Can you work these out from the model? Positions are in its coordinate system, mm. Face numbers are marked on the shaded views. A direction names the side the tool comes from. Give positions to 0.01 mm unless a question says otherwise; leave off trailing zeros. Loops run counter-clockwise (first coordinate to the right, second up) from the corner with the lowest first, then second, coordinate; pieces in that order, holes last. Notation, with made-up numbers: (8.5, 19.5) - (56.5, 19.5) arc R22 ccw to (56.5, 28.5) - close; hole circle Ø7 at (-12, 59.5). An arc over 180 degrees is marked (long way). Answer as a JSON object with one key per item and string values.
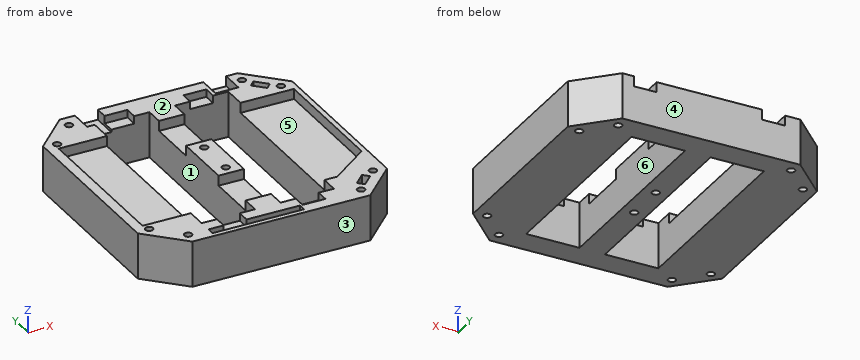
```python
from build123d import *

# Parameters (mm, degrees)
PAD_DEPTH       = 18
SKETCH001_R     = 1.5
POCKET_DEPTH    = 18.001
SKETCH002_W     = 21
SKETCH002_H     = 78
POCKET001_DEPTH = 18.001
SKETCH003_W     = 9
SKETCH003_H     = 88
POCKET002_DEPTH = 3
SKETCH004_W     = 12
SKETCH004_H     = 20
SKETCH004_W_2   = 19
SKETCH004_H_2   = 62
SKETCH004_W_3   = 9
SKETCH004_H_3   = 9
SKETCH004_W_4   = 36
SKETCH004_H_4   = 3
POCKET003_DEPTH = 4
SKETCH005_W     = 6
SKETCH005_H     = 1
POCKET004_DEPTH = 4


with BuildPart() as part:
    # Sketch → Pad (new body)
    with BuildSketch(Plane.XY):
        Polygon((-49, 35), (-35, 49), (35, 49), (49, 35), (49, -35), (35, -49), (-35, -49), (-49, -35), align=None)
    extrude(amount=PAD_DEPTH)

    # Sketch001 (on DatumPlane) → Pocket (cut, through all)
    with BuildSketch(Plane.XY.offset(18)):
        with Locations((-34, 44)):
            Circle(SKETCH001_R)
        with Locations((34, 44)):
            Circle(SKETCH001_R)
        with Locations((44, 34)):
            Circle(SKETCH001_R)
        with Locations((-44, 34)):
            Circle(SKETCH001_R)
        with Locations((-44, -34)):
            Circle(SKETCH001_R)
        with Locations((-34, -44)):
            Circle(SKETCH001_R)
        with Locations((34, -44)):
            Circle(SKETCH001_R)
        with Locations((44, -34)):
            Circle(SKETCH001_R)
        with Locations((0, 8)):
            Circle(SKETCH001_R)
        with Locations((0, -8)):
            Circle(SKETCH001_R)
    extrude(amount=-POCKET_DEPTH, mode=Mode.SUBTRACT)

    # Sketch002 (on DatumPlane) → Pocket001 (cut, through all)
    with BuildSketch(Plane.XY.offset(18)):
        with Locations((-15.5, 0)):
            Rectangle(SKETCH002_W, SKETCH002_H)
        with Locations((15.5, 0)):
            Rectangle(SKETCH002_W, SKETCH002_H)
    extrude(amount=-POCKET001_DEPTH, mode=Mode.SUBTRACT)

    # Sketch003 (on DatumPlane) → Pocket002 (cut)
    with BuildSketch(Plane.XY.offset(18)):
        with Locations((-15.5, 0)):
            Rectangle(SKETCH003_W, SKETCH003_H)
        with Locations((15.5, 0)):
            Rectangle(SKETCH003_W, SKETCH003_H)
    extrude(amount=-POCKET002_DEPTH, mode=Mode.SUBTRACT)

    # Sketch004 (on DatumPlane) → Pocket003 (cut)
    with BuildSketch(Plane.XY.offset(18)):
        with Locations((0, 22)):
            Rectangle(SKETCH004_W, SKETCH004_H)
        with Locations((0, -22)):
            Rectangle(SKETCH004_W, SKETCH004_H)
        with Locations((-35.5, 0)):
            Rectangle(SKETCH004_W_2, SKETCH004_H_2)
        with Locations((-24.5, 44.5)):
            Rectangle(SKETCH004_W_3, SKETCH004_H_3)
        with Locations((26, 44.5)):
            Rectangle(SKETCH004_W_3, SKETCH004_H_3)
        Polygon((37.050253, 41.292893), (41.292893, 37.050253), (39.171573, 34.928932), (34.928932, 39.171573), align=None)
        Polygon((34.928932, -39.171573), (37.050253, -41.292893), (41.292893, -37.050253), (39.171573, -34.928932), align=None)
        with Locations((-8, -45.5)):
            Rectangle(SKETCH004_W_4, SKETCH004_H_4)
        Polygon((47, 30), (26, 30), (26, -32), (31, -32), (47, -20), align=None)
    extrude(amount=-POCKET003_DEPTH, mode=Mode.SUBTRACT)

    # Sketch005 (on DatumPlane) → Pocket004 (cut)
    with BuildSketch(Plane.XY.offset(18)):
        with Locations((-23, 39.5)):
            Rectangle(SKETCH005_W, SKETCH005_H)
    extrude(amount=-POCKET004_DEPTH, mode=Mode.SUBTRACT)


solid = part.part
```
1) I need wall thicknesses on L1, parallel to Y at x = 0, z = 4.75; L2, parallel to X at y = -5.5, z = 6.5; L3, parallel to Y at x = 12, z = 7.25. Which ranges of each line are inside material? Lowest first, please.
Check sheet entries:
{"L1": "-49 to -9.5, -6.5 to 6.5, 9.5 to 49", "L2": "-49 to -26, -5 to 5, 26 to 49", "L3": "-49 to -39, 39 to 49"}
2) Imagine slicing it at B-B on x = -9. Write out the boundary of the cut face in (y, z).
Check sheet entries:
{"outline": "(-49, 0) - (-39, 0) - (-39, 18) - (-44, 18) - (-44, 14) - (-47, 14) - (-47, 18) - (-49, 18) - close; (39, 0) - (49, 0) - (49, 18) - (39, 18) - close"}
3) I'm going to push flat-ended pins straight in: P1, Ø3, axis at x = 28.5, z = 16.5, coming from the +Y side; P2, Ø5, axis at x = -35.5, y = -23, coming from the +Z side; P3, Ø3.5, axis at y = -45.5, z = 15.5, coming from the -X side. Where does each tip first touch, or does it pass through?
Check sheet entries:
{"P1": "y = 40", "P2": "z = 14", "P3": "x = -40.25"}
4) Which directions (+Z, -Z, +X, -X, +Y, -Y) give clear straight access to the entire face, cutting with the end or side of a thin tool? Please do the marked faces 4, 5 and 6.
Check sheet entries:
{"face 4": "+Z, -Z, +X, -X, +Y", "face 5": "+Z", "face 6": "+Z, -Z"}
5) Imagine slicing it at C-C on x = 44. Write out the boundary of the cut face in (y, z).
Check sheet entries:
{"outline": "(-40, 0) - (-35.5, 0) - (-35.5, 18) - (-40, 18) - close; (-32.5, 0) - (32.5, 0) - (32.5, 18) - (30, 18) - (30, 14) - (-22.25, 14) - (-22.25, 18) - (-32.5, 18) - close; (35.5, 0) - (40, 0) - (40, 18) - (35.5, 18) - close"}
6) Imagine slicing it at A-A on y = -3. Write out the boundary of the cut face in (x, z), and give its area (3 significant figures).
Check sheet entries:
{"outline": "(-49, 0) - (-26, 0) - (-26, 14) - (-45, 14) - (-45, 18) - (-49, 18) - close; (-5, 0) - (5, 0) - (5, 18) - (-5, 18) - close; (26, 0) - (49, 0) - (49, 18) - (47, 18) - (47, 14) - (26, 14) - close", "area": "848 mm2"}
7) Imagine slicing it at D-D on z = 9.5. Give the number of separate pieces and of enclosed holes in the cut face, and give its area (3 significant figures).
Check sheet entries:
{"separate pieces": "1", "enclosed holes": "12", "area": "5,870 mm2"}
8) If we mould it in two halves opening along Y, with no side actions, what happens to the marked faces 1, 2 and 3? For each: released by +Y, released by -Y, zero draft, split by the parting line, or undercut.
Check sheet entries:
{"face 1": "undercut", "face 2": "zero draft", "face 3": "released by -Y"}
